Work out the finished part from the listing and answer in its coordinate system (mm). Give positions to 0.01 mm unless a question says otherwise; leave off trailing zeros. Loops run counter-clockwise (first coordinate to the right, second up) from the corner with the lowest first, then second, coordinate; pieces in that order, holes last. Notation, with made-up numbers: (56, 5) - (80, 5) arc R12 cw to (80, 24) - close; hole circle Ø1 at (-24, 81). An arc over 180 degrees is marked (long way). One line per question, with ' | ' between items.
from build123d import *

# Parameters (mm, degrees)
SKETCH_2_W          = 75
SKETCH_2_H          = 613
EXTRUDE_1_DEPTH     = 4
SKETCH_7_W          = 23.197141887
SKETCH_7_H          = 202.515498828
CUT_EXTRUDE_2_DEPTH = 5
FILLET_1_R          = 3
SKETCH_8_R          = 1.75
CUT_EXTRUDE_3_DEPTH = 5
SKETCH_9_R          = 2.5
CUT_EXTRUDE_4_DEPTH = 5
SKETCH_10_R         = 2.5
CUT_EXTRUDE_5_DEPTH = 5


with BuildPart() as part:
    # 草图2 → 凸台-拉伸1 (new body)
    with BuildSketch(Plane.XY):
        with Locations((37.5, -306.5)):
            Rectangle(SKETCH_2_W, SKETCH_2_H)
    extrude(amount=EXTRUDE_1_DEPTH)

    # 草图7 → 切除-拉伸2 (cut, through all)
    with BuildSketch(Plane(origin=(0, 0, 0), x_dir=(-1, 0, 0), z_dir=(0, 0, -1))):
        with Locations((-63.401429057, -101.257749414)):
            Rectangle(SKETCH_7_W, SKETCH_7_H)
    extrude(amount=-CUT_EXTRUDE_2_DEPTH, mode=Mode.SUBTRACT)

    # 圆角1
    fillet_1_edges = [part.edges().sort_by_distance(p)[0] for p in [
        (75, -202.515498828, 2),
        (51.802858113, 0, 2),
        (51.802858113, -202.515498828, 2),
    ]]
    fillet(fillet_1_edges, radius=FILLET_1_R)

    # 草图8 → 切除-拉伸3 (cut, through all)
    with BuildSketch(Plane(origin=(0, 0, 0), x_dir=(-1, 0, 0), z_dir=(0, 0, -1))):
        with Locations((-48.75, -17.5)):
            Circle(SKETCH_8_R)
        with Locations((-48.75, -37.5)):
            Circle(SKETCH_8_R)
        with Locations((-48.75, -57.5)):
            Circle(SKETCH_8_R)
        with Locations((-48.75, -77.5)):
            Circle(SKETCH_8_R)
        with Locations((-48.75, -97.5)):
            Circle(SKETCH_8_R)
        with Locations((-48.75, -117.5)):
            Circle(SKETCH_8_R)
        with Locations((-48.75, -137.5)):
            Circle(SKETCH_8_R)
        with Locations((-48.75, -157.5)):
            Circle(SKETCH_8_R)
        with Locations((-48.75, -177.5)):
            Circle(SKETCH_8_R)
        with Locations((-48.75, -197.5)):
            Circle(SKETCH_8_R)
        with Locations((-48.75, -217.5)):
            Circle(SKETCH_8_R)
        with Locations((-48.75, -237.5)):
            Circle(SKETCH_8_R)
        with Locations((-48.75, -257.5)):
            Circle(SKETCH_8_R)
        with Locations((-48.75, -277.5)):
            Circle(SKETCH_8_R)
        with Locations((-48.75, -297.5)):
            Circle(SKETCH_8_R)
        with Locations((-48.75, -317.5)):
            Circle(SKETCH_8_R)
        with Locations((-48.75, -337.5)):
            Circle(SKETCH_8_R)
        with Locations((-48.75, -357.5)):
            Circle(SKETCH_8_R)
        with Locations((-48.75, -377.5)):
            Circle(SKETCH_8_R)
        with Locations((-48.75, -397.5)):
            Circle(SKETCH_8_R)
        with Locations((-48.75, -417.5)):
            Circle(SKETCH_8_R)
        with Locations((-48.75, -437.5)):
            Circle(SKETCH_8_R)
        with Locations((-48.75, -457.5)):
            Circle(SKETCH_8_R)
        with Locations((-48.75, -477.5)):
            Circle(SKETCH_8_R)
        with Locations((-48.75, -497.5)):
            Circle(SKETCH_8_R)
        with Locations((-48.75, -517.5)):
            Circle(SKETCH_8_R)
        with Locations((-48.75, -537.5)):
            Circle(SKETCH_8_R)
        with Locations((-48.75, -557.5)):
            Circle(SKETCH_8_R)
        with Locations((-48.75, -577.5)):
            Circle(SKETCH_8_R)
        with Locations((-48.75, -597.5)):
            Circle(SKETCH_8_R)
    extrude(amount=-CUT_EXTRUDE_3_DEPTH, mode=Mode.SUBTRACT)

    # 草图9 → 切除-拉伸4 (cut, through all)
    with BuildSketch(Plane.XY.offset(4)):
        with Locations((11.75, -593)):
            Circle(SKETCH_9_R)
        with Locations((11.75, -563)):
            Circle(SKETCH_9_R)
        with Locations((11.75, -533)):
            Circle(SKETCH_9_R)
        with Locations((11.75, -503)):
            Circle(SKETCH_9_R)
        with Locations((11.75, -473)):
            Circle(SKETCH_9_R)
        with Locations((11.75, -443)):
            Circle(SKETCH_9_R)
        with Locations((11.75, -413)):
            Circle(SKETCH_9_R)
        with Locations((11.75, -383)):
            Circle(SKETCH_9_R)
        with Locations((11.75, -353)):
            Circle(SKETCH_9_R)
        with Locations((11.75, -323)):
            Circle(SKETCH_9_R)
        with Locations((11.75, -293)):
            Circle(SKETCH_9_R)
        with Locations((11.75, -263)):
            Circle(SKETCH_9_R)
        with Locations((11.75, -233)):
            Circle(SKETCH_9_R)
        with Locations((11.75, -203)):
            Circle(SKETCH_9_R)
        with Locations((11.75, -173)):
            Circle(SKETCH_9_R)
        with Locations((11.75, -143)):
            Circle(SKETCH_9_R)
        with Locations((11.75, -113)):
            Circle(SKETCH_9_R)
        with Locations((11.75, -83)):
            Circle(SKETCH_9_R)
        with Locations((11.75, -53)):
            Circle(SKETCH_9_R)
        with Locations((11.75, -23)):
            Circle(SKETCH_9_R)
    extrude(amount=-CUT_EXTRUDE_4_DEPTH, mode=Mode.SUBTRACT)

    # 草图10 → 切除-拉伸5 (cut, through all)
    with BuildSketch(Plane.XY.offset(4)):
        with Locations((63.25, -605.950596653)):
            Circle(SKETCH_10_R)
        with Locations((63.25, -515.950596653)):
            Circle(SKETCH_10_R)
        with Locations((63.25, -425.950596653)):
            Circle(SKETCH_10_R)
        with Locations((63.25, -335.950596653)):
            Circle(SKETCH_10_R)
        with Locations((63.25, -245.950596653)):
            Circle(SKETCH_10_R)
    extrude(amount=-CUT_EXTRUDE_5_DEPTH, mode=Mode.SUBTRACT)


solid = part.part
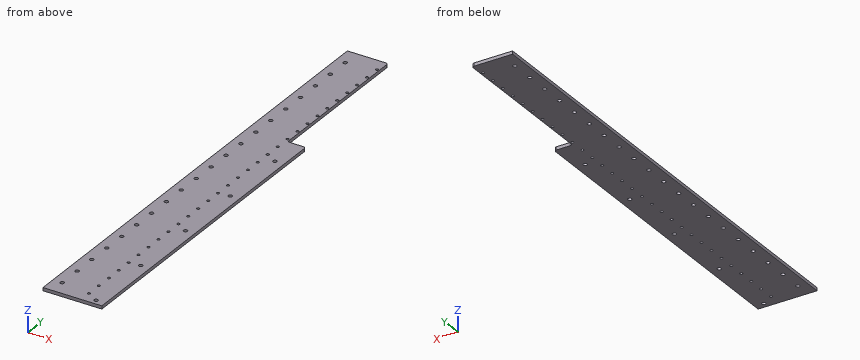
1. Consider L1, parallel to X at y = -233, z = 1.65; L2, parallel to X at y = -277.5, z = 1.3; L3, parallel to X at y = -517.5, z = 1.75. Determine where each line is inside the solid, lowest interval first.
Evaluation:
L1: 0 to 9.25, 14.25 to 75 | L2: 0 to 47, 50.5 to 75 | L3: 0 to 47, 50.5 to 61.29, 65.21 to 75
2. Find section A-A on y = -66. Write down the section's boundary in (x, z), then the cut area to 3 significant figures.
Evaluation:
outline: (0, 0) - (51.8, 0) - (51.8, 4) - (0, 4) - close | area: 207 mm2
3. Flat-ended cylindrical pins translate along their axes: pin 1 (2 mm diameter, centred on y = -200.5, z = 1.5, fed in from +X); pin 2 (6.5 mm diameter, centred on x = 11.75, y = -533, fed in from -Z). Find the tip coordinate at first contact, or state that the pin passes through.
Evaluation:
pin 1: x = 52.55 | pin 2: z = 0
4. Find section B-B on z = 2.05. State how many separate pieces and enclosed holes the cut face has, then the cut area to 3 significant figures.
Evaluation:
separate pieces: 1 | enclosed holes: 55 | area: 40,500 mm2
